from build123d import *

# Parameters (mm, degrees)
SKETCH1_R           = 12
SKETCH1_R_2         = 6
BOSS_EXTRUDE1_DEPTH = 6
SKETCH2_R           = 10.5
SKETCH2_R_2         = 7.5
CUT_EXTRUDE1_DEPTH  = 0.3
CUT_EXTRUDE2_START  = -5.5
SKETCH2_2_R         = 10.5
SKETCH2_2_R_2       = 7.5
CUT_EXTRUDE2_DEPTH  = 0.5
FILLET1_R           = 0.15


with BuildPart() as part:
    # Sketch1 → Boss-Extrude1 (new body)
    with BuildSketch(Plane.XY):
        Circle(SKETCH1_R)
        Circle(SKETCH1_R_2, mode=Mode.SUBTRACT)
    extrude(amount=BOSS_EXTRUDE1_DEPTH)

    # Sketch2 → Cut-Extrude1 (cut)
    with BuildSketch(Plane.XY.offset(6)):
        Circle(SKETCH2_R)
        Circle(SKETCH2_R_2, mode=Mode.SUBTRACT)
    extrude(amount=-CUT_EXTRUDE1_DEPTH, mode=Mode.SUBTRACT)

    # Sketch2<2> → Cut-Extrude2 (cut)
    with BuildSketch(Plane.XY.offset(6).offset(CUT_EXTRUDE2_START)):
        Circle(SKETCH2_2_R)
        Circle(SKETCH2_2_R_2, mode=Mode.SUBTRACT)
    extrude(amount=-CUT_EXTRUDE2_DEPTH, mode=Mode.SUBTRACT)

    # Fillet1
    fillet1_edges = [part.edges().sort_by_distance(p)[0] for p in [
        (-12, 0, 0),
        (-12, 0, 6),
        (-6, 0, 0),
        (-6, 0, 6),
    ]]
    fillet(fillet1_edges, radius=FILLET1_R)


solid = part.part
Model file for the job. Use its own axes, mm. A direction names the side the tool comes from. Round coordinates to 2 decimals unless told otherwise and drop trailing zeros. Loops run counter-clockwise (first coordinate to the right, second up) from the corner with the lowest first, then second, coordinate; pieces in that order, holes last. Notation, with made-up numbers: (51, 46) -> (56, 46) arc R18 cw to (56, 59) -> close; hole circle Ø4 at (34, 10). An arc over 180 degrees is marked (long way). Answer as CSV lines item,"result". Start each with the question number.
1) Slice it at C-C (z = 3.55). List the corners of the cut face in (x, y), plus the area to 3 significant figures.
2) Pin check, flat tips, straight feed: P1, Ø1.5, axis at x = -6.5, z = 2.5, coming from the -Y side; P2, Ø2, axis at x = -4.5, z = 1, coming from the +Y side. Stop position of each tip, or through.
3) Mould opens along Y. For faces 1 (the face through (-1.63, -7.32, 5.85)), 2 (the face through (-11.99, 0.53, 2.96)), 3 (the face through (-6, 3, 0)) say: +Y half, -Y half, draft (parallel to the pull), parting line (faces both ways), or undercut.
4) Probe line 1 along Y through (x, z) = (0, 5.8); line 2 along Y through (x, z) = (0, 2.4); line 3 along Z through (x, y) = (-5.25, -6.5). List the from-to ranges inside material, lowest first.
5) Tool access for faces 4 (the face through (5, -7, 5.7)), 5 (the face through (-7.493, 0.33, 0.254)), 6 (the face through (-6, 3, 6)): list every direction of +Z, -Z, +X, -X, +Y, -Y with a clear straight run to the whole face (end or side of a thin tool).
Filled in:
1,outline,"circle Ø24 at (0, 0); hole circle Ø12 at (0, 0)"
1,area,"339 mm2"
2,P1,"stops at y = -10.53"
2,P2,"stops at y = 11.48"
3,face 1,"undercut"
3,face 2,"parting line"
3,face 3,"draft"
4,line 1,"y = -12 to -10.5, -7.5 to -6, 6 to 7.5, 10.5 to 12"
4,line 2,"y = -12 to -6, 6 to 12"
4,line 3,"z = 0.5 to 5.7"
5,face 4,"+Z"
5,face 5,"-Z"
5,face 6,"+Z, +X, -X, +Y, -Y"
